Input: dimensioned drawing with shaded views. Units: mm. Origin: part minimum x, y, z. A direction names the side the tool comes from. Round coordinates to 2 decimals unless told otherwise and drop trailing zeros. Loops run counter-clockwise (first coordinate to the right, second up) from the corner with the lowest first, then second, coordinate; pieces in that order, holes last. Notation, with made-up numbers: M 47,66.25 L 70,66.25 A14 cw 70,90.25 Z; hole C 13.5,37.5 d5. An arc over 180 degrees is marked long. Use one line per item in the form item = value. Start each with the question number.
Q1. Section query B-B, the plane x = 111.76. Output: boundary loops of the cut face in (y, z), and give its area (3 significant figures).
Q2. Section query D-D, the plane x = 25.4. Output: boundary loops of the cut face in (y, z), and give its area (3 significant figures).
Q3. Ray query, line 1 along Y through (x, z) = (25.4, 0.7); line 2 along Y through (x, z) = (47, 24); line 3 along Z through (x, y) = (98, 6). Return the intervals inside material, ascending.
Q4. Section query C-C, the plane z = 5. Output: boundary loops of the cut face in (x, y).
Q5. Mould query, pull axis Y, two halves, no side actions, for the marked faces 3, 4 and 5. Classes: pulls with the +Y half, pulls with the -Y half, needs draft (parallel to the pull), parting line crosses it, or undercut.
Q6. Section query A-A, the plane z = 19.05. State how many separate pieces and enclosed holes the cut face has, and give its area (3 significant figures).
Q7. Access query for the marked faces 1 and 2. Directions: +Z, -Z, +X, -X, +Y, -Y. A direction counts if a zero-diameter tool reaches every point of the face in a straight line with its end or side. Return the directions, or none.
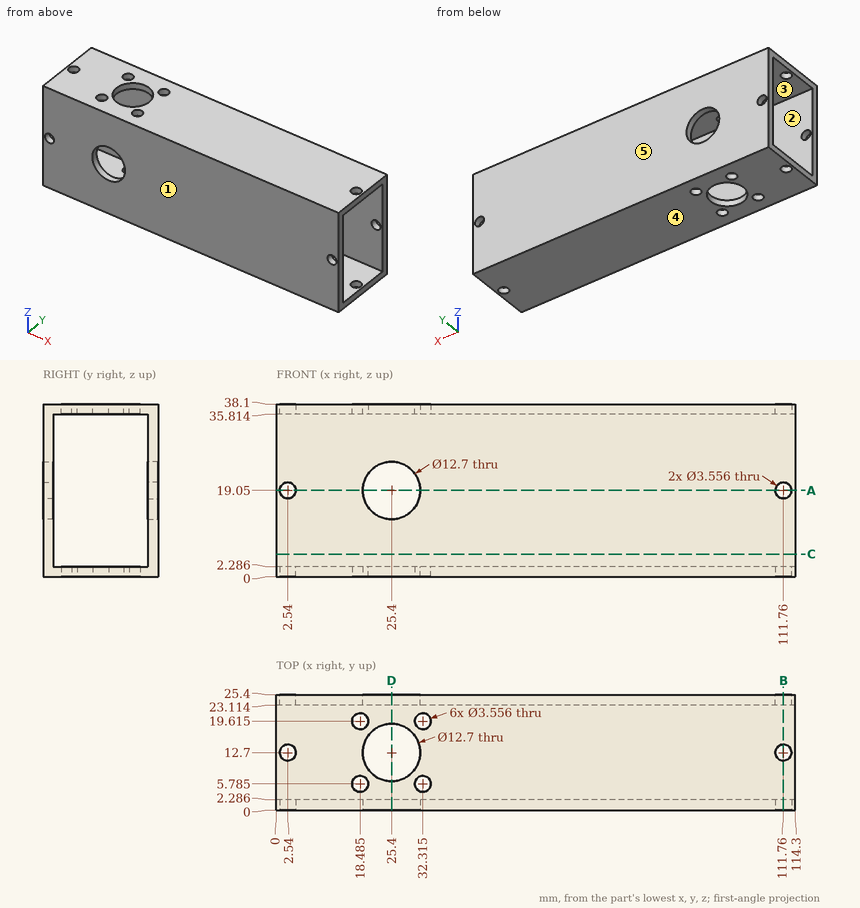
Results found:
q1.outline = M 0,0 L 10.92,0 L 10.92,2.29 L 2.29,2.29 L 2.29,17.27 L 0,17.27 Z; M 0,20.83 L 2.29,20.83 L 2.29,35.81 L 10.92,35.81 L 10.92,38.1 L 0,38.1 Z; M 14.48,0 L 25.4,0 L 25.4,17.27 L 23.11,17.27 L 23.11,2.29 L 14.48,2.29 Z; M 14.48,35.81 L 23.11,35.81 L 23.11,20.83 L 25.4,20.83 L 25.4,38.1 L 14.48,38.1 Z
q1.area = 237 mm²
q2.outline = M 0,0 L 6.35,0 L 6.35,2.29 L 2.29,2.29 L 2.29,12.7 L 0,12.7 Z; M 0,25.4 L 2.29,25.4 L 2.29,35.81 L 6.35,35.81 L 6.35,38.1 L 0,38.1 Z; M 19.05,0 L 25.4,0 L 25.4,12.7 L 23.11,12.7 L 23.11,2.29 L 19.05,2.29 Z; M 19.05,35.81 L 23.11,35.81 L 23.11,25.4 L 25.4,25.4 L 25.4,38.1 L 19.05,38.1 Z
q2.area = 153 mm²
q3.line_1 = 0 to 6.35, 19.05 to 25.4
q3.line_2 = 0 to 2.29, 23.11 to 25.4
q3.line_3 = 0 to 2.29, 35.81 to 38.1
q4.outline = M 0,0 L 114.3,0 L 114.3,2.29 L 0,2.29 Z; M 0,23.11 L 114.3,23.11 L 114.3,25.4 L 0,25.4 Z
q5.face_3 = undercut
q5.face_4 = needs draft
q5.face_5 = pulls with the +Y half
q6.separate_pieces = 8
q6.enclosed_holes = 0
q6.area = 432 mm²
q7.face_1 = +Z, -Z, +X, -X, -Y
q7.face_2 = +X, -X
